```python
from build123d import *

# Parameters (mm, degrees)
F0_W     = 4.5
F0_H     = 1.1
F1_DEPTH = 0.6
F2_W     = 4.5
F2_H     = 2.2
F3_DEPTH = 1.6
F4_R     = 1.09999
F5_R     = 0.5
F6_DEPTH = 25


# Not quite as in the source:
# - a fillet or chamfer is up to 0.001 mm smaller than in the source, because OpenCascade refuses the exact size


with BuildPart() as f1:
    # F0 (on Top) → F1 (new body)
    with BuildSketch(Plane.XY):
        with Locations((12.75, 2.75)):
            Rectangle(F0_W, F0_H)
        with Locations((12.75, 3.85)):
            Rectangle(F0_W, F0_H)
        with BuildLine():
            Line((10.1278736967, 2.2), (10.5, 2.2))
            Line((10.5, 2.2), (10.5, 3.3))
            Line((10.5, 3.3), (9.5, 3.3))
            Line((9.5, 3.3), (9.5, 2.1397182935))
            ThreePointArc((9.5, 2.1397182935), (9.8124932664, 2.1848950035), (10.1278736967, 2.2))
        make_face()
        with BuildLine():
            Line((9.5, 3.3), (10.5, 3.3))
            Line((10.5, 3.3), (10.5, 4.4))
            Line((10.5, 4.4), (10.1278736967, 4.4))
            ThreePointArc((10.1278736967, 4.4), (9.8124932664, 4.4151049965), (9.5, 4.4602817065))
            Line((9.5, 4.4602817065), (9.5, 3.3))
        make_face()
        with BuildLine():
            Line((9.5, 2.1397182935), (9.5, 3.3))
            Line((9.5, 3.3), (9.5, 4.4602817065))
            ThreePointArc((9.5, 4.4602817065), (9.2040660975, 4.5319438894), (8.9159970588, 4.6305774135))
            Line((8.9159970588, 4.6305774135), (4.5118766379, 6.3694225865))
            ThreePointArc((4.5118766379, 6.3694225865), (3.9168085053, 6.5418431899), (3.3, 6.6))
            Line((3.3, 6.6), (3.3, 5.15))
            ThreePointArc((3.3, 5.15), (4.6081475452, 4.6081475452), (5.15, 3.3))
            ThreePointArc((5.15, 3.3), (4.6081475452, 1.9918524548), (3.3, 1.45))
            Line((3.3, 1.45), (3.3, 0))
            ThreePointArc((3.3, 0), (3.9168085053, 0.0581568101), (4.5118766379, 0.2305774135))
            Line((4.5118766379, 0.2305774135), (8.9159970588, 1.9694225865))
            ThreePointArc((8.9159970588, 1.9694225865), (9.2040660975, 2.0680561106), (9.5, 2.1397182935))
        make_face()
        with BuildLine():
            ThreePointArc((0, 3.3), (0.9665476221, 0.9665476221), (3.3, 0))
            Line((3.3, 0), (3.3, 1.45))
            ThreePointArc((3.3, 1.45), (1.45, 3.3), (3.3, 5.15))
            Line((3.3, 5.15), (3.3, 6.6))
            ThreePointArc((3.3, 6.6), (0.9665476221, 5.6334523779), (0, 3.3))
        make_face()
    extrude(amount=F1_DEPTH)

    # F2 (on face) → F3 (join)
    with BuildSketch(Plane.XY.offset(0.6)):
        with Locations((12.75, 3.3)):
            Rectangle(F2_W, F2_H)
    extrude(amount=F3_DEPTH)

    # F4 (radius 1.1 in the source; OpenCascade refuses exactly that, so slightly less here)
    f4_edges = [f1.edges().sort_by_distance(p)[0] for p in [
        (12.75, 2.2, 2.2),
        (12.75, 4.4, 2.2),
    ]]
    fillet(f4_edges, radius=F4_R)

    # F5 (on face) → F6 (cut)
    with BuildSketch(Plane.YZ.offset(15)):
        with Locations((3.3, 1.1)):
            Circle(F5_R)
    extrude(amount=-F6_DEPTH, mode=Mode.SUBTRACT)


solid = f1.part
```
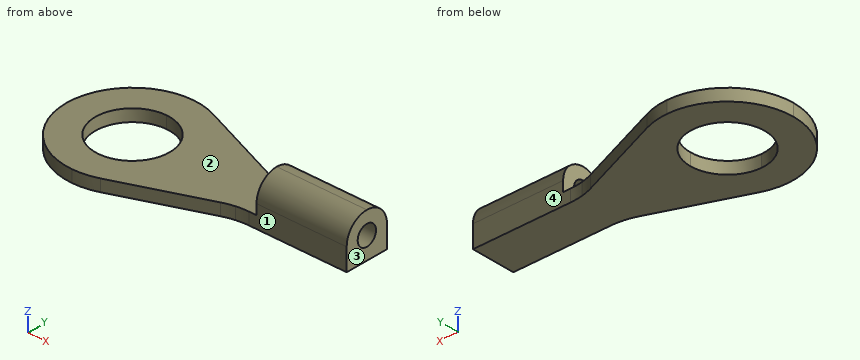
Work out the finished part from the listing and answer in its coordinate system (mm). Face numbers are marked on the shaded views. A direction names the side the tool comes from. Round coordinates to 2 decimals unless told otherwise and drop trailing zeros. Write each loop counter-clockwise with the first axis right and the second up, starting at its lowest first coordinate (ties: lowest second). Pieces come first, ordered by that corner, then holes. Notation, with made-up numbers: (16, 44) -> (50, 44) arc R22 ccw to (50, 53) -> close; hole circle Ø11 at (-31.5, 64). An arc over 180 degrees is marked (long way). Write each question's results on one line, items separated by ' | '.
Q1. Section A-A, the plane y = 3.5 is taken. Write down the section's boundary in (x, z), then the cut area to 3 significant figures.
Data:
outline: (0.01, 0) -> (1.46, 0) -> (1.46, 0.6) -> (0.01, 0.6) -> close; (5.14, 0) -> (15, 0) -> (15, 0.64) -> (10.5, 0.64) -> (10.5, 0.6) -> (5.14, 0.6) -> close; (10.5, 1.56) -> (15, 1.56) -> (15, 2.18) -> (10.5, 2.18) -> close | area: 9.78 mm^2
Q2. Straight lines are drawn through the part: line 1 along Y through (x, z) = (13.4, 1.1); line 2 along X through (y, z) = (3.25, 0.5); line 3 along Z through (x, y) = (12.25, 3.3). For each, find the intervals that lie inside material, in ascending order. Write a range as [from, to].
Data:
line 1: [2.2, 2.8], [3.8, 4.4] | line 2: [0, 1.45], [5.15, 15] | line 3: [0, 0.6], [1.6, 2.2]
Q3. Section C-C, the plane z = 0.75 is taken. Write down the section's boundary in (x, y), then the cut area to 3 significant figures.
Data:
outline: (10.5, 2.2) -> (15, 2.2) -> (15, 2.94) -> (10.5, 2.94) -> close; (10.5, 3.66) -> (15, 3.66) -> (15, 4.4) -> (10.5, 4.4) -> close | area: 6.69 mm^2
Q4. Section D-D, the plane y = 2.5 is taken. Write down the section's boundary in (x, z).
Data:
outline: (0.1, 0) -> (1.63, 0) -> (1.63, 0.6) -> (0.1, 0.6) -> close; (4.97, 0) -> (15, 0) -> (15, 1.85) -> (10.5, 1.85) -> (10.5, 0.6) -> (4.97, 0.6) -> close
Q5. Which of the six approach directions +Z, -Z, +X, -X, +Y, -Y give full straight-line access (tool end or side, diameter ignored) to the marked faces 1, 2, 3 and 4?
Data:
face 1: +Z, -Z, +X, -Y | face 2: +Z, -X, +Y, -Y | face 3: +Z, -Z, +X, +Y, -Y | face 4: +Z, -Z, +X, +Y
Q6. Flat-ended cylindrical pins translate along their axes: P1, Ø0.5, axis at y = 3, z = 1.5, coming from the -X side; P2, Ø2, axis at x = 5.5, y = 4, coming from the +Z side; P3, Ø0.6, axis at x = 13.5, z = 0.5, coming from the +Y side. Find the tip coordinate at first contact, or state that the pin passes through.
Data:
P1: x = 10.5 | P2: z = 0.6 | P3: y = 4.4
